Read the model definition and answer for the solid it produces. Units are mm, in the model's axes. Face numbers are marked on the shaded views. Round coordinates to 2 decimals unless told otherwise and drop trailing zeros. Loops run counter-clockwise (first coordinate to the right, second up) from the corner with the lowest first, then second, coordinate; pieces in that order, holes last. Notation, with made-up numbers: M 82.5,-30.75 L 91.5,-30.75 A37 ccw 91.5,5.25 Z; hole C 70.25,65.25 d1. An arc over 180 degrees is marked long. Write each question's results on one line, items separated by ' | '.
```python
from build123d import *

# Parameters (mm, degrees)
F0_R        = 1.075
F3_DEPTH    = 1.2
F2_W        = 15
F2_H        = 1.2
F4_DEPTH    = 10
F1_W        = 15
F1_H        = 1.2
F5_DEPTH    = 12
F6_T1_DEPTH = 38.762491
F7_R        = 2
F8_R        = 1
F10_D       = 3


# Not quite as in the source:
# - a fillet or chamfer that OpenCascade refuses, or shapes differently, is made with other operations: its cross-section is extruded or revolved along the edge and cut away or added


with BuildPart() as f3:
    # F0 (on Top) → F3 (new body)
    with BuildSketch(Plane.XY):
        Polygon((-15, 0), (0, 0), (0, 60), (-15, 60), (-15, 58.8), (-11, 58.8), (-10.4650629229, 8.8028616587), (-15, 7), align=None)
        with Locations((-2, 10)):
            Circle(F0_R, mode=Mode.SUBTRACT)
        with Locations((-2, 50)):
            Circle(F0_R, mode=Mode.SUBTRACT)
    extrude(amount=F3_DEPTH)

    # F2 (on face) → F4 (join)
    with BuildSketch(Plane.XY):
        with Locations((-7.5, 0.6)):
            Rectangle(F2_W, F2_H)
    extrude(amount=F4_DEPTH)

    # F1 (on face) → F5 (join)
    with BuildSketch(Plane.XY):
        with Locations((-7.5, 59.3886146865)):
            Rectangle(F1_W, F1_H)
    extrude(amount=F5_DEPTH)

    # F6: fillet of radius 7.5124982 on 2 edges, made by hand

    # F6_s2 → F6_t1 (cut)
    with BuildSketch(Plane.XZ.offset(-78.7698601865)):
        with BuildLine():
            ThreePointArc((0, 4.4875018), (-2.2003597791, 9.7996402209), (-7.5124982, 12))
            Line((-7.5124982, 12), (0, 12))
            Line((0, 12), (0, 4.4875018))
        make_face()
        with BuildLine():
            ThreePointArc((-15, 4.4875018), (-12.7996402209, 9.7996402209), (-7.4875018, 12))
            Line((-7.4875018, 12), (-15, 12))
            Line((-15, 12), (-15, 4.4875018))
        make_face()
    extrude(amount=F6_T1_DEPTH, mode=Mode.SUBTRACT)

    # F7
    f7_edges = [f3.edges().sort_by_distance(p)[0] for p in [
        (0, 0.6, 10),
        (-15, 0.6, 10),
    ]]
    fillet(f7_edges, radius=F7_R)

    # F8
    f8_edges = [f3.edges().sort_by_distance(p)[0] for p in [
        (-7.5, 0, 0),
        (-7.5, 60, 0),
    ]]
    fillet(f8_edges, radius=F8_R)

    # F10 (through all)
    with Locations(Plane.XZ):
        with Locations((-7.506201975, 4.490504507)):
            Hole(F10_D / 2)


solid = f3.part
```
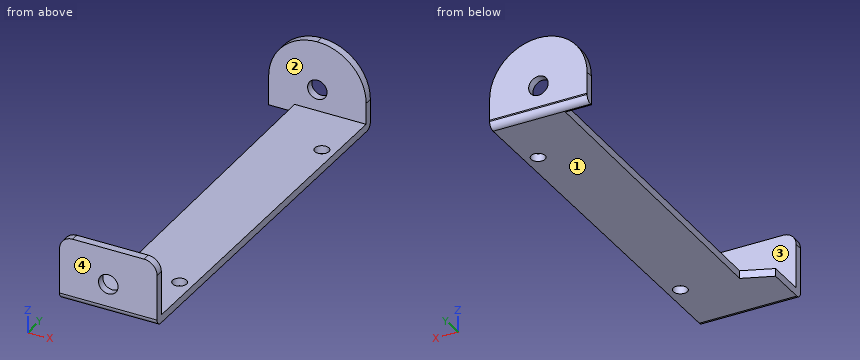
1. Given P1, Ø1, axis at x = -10.5, y = 24, coming from the +Z side; P2, Ø1, axis at x = -10, y = 1, coming from the +Z side; P3, Ø2.5, axis at x = -7.51, z = 4.49, coming from the -Y side; P4, Ø1, axis at x = -6.5, z = 5.5, coming from the +Y side, each flat-ended and moving along its own axis, determine where each tip first touches the part or whether it passes through.
Completed:
P1: stops at z = 1.2 | P2: stops at z = 10 | P3: passes through | P4: stops at y = 59.99
2. Find the intervals of material crossed by L1, parallel to Y at x = -2.75, z = 3; L2, parallel to Y at x = -2, z = 0.8 (3 decimals); L3, parallel to Y at x = -2, z = 0.4 (3 decimals), in increasing order.
Completed:
L1: y = 0 to 1.2, 58.79 to 59.99 | L2: y = 0.02 to 8.925, 11.075 to 48.925, 51.075 to 59.98 | L3: y = 0.2 to 8.925, 11.075 to 48.925, 51.075 to 59.8
3. Determine the mould class of the marked faces 1, 2, 3 and 4 for opening direction Y: released by +Y, released by -Y, zero draft, split by the parting line, or undercut.
Completed:
face 1: zero draft | face 2: undercut | face 3: undercut | face 4: released by -Y
4. Find section A-A, the plane z = 1.75. Give the vertices of the cut face in (x, y).
Completed:
outline: M -15,0 L 0,0 L 0,1.2 L -15,1.2 Z; M -15,58.79 L 0,58.79 L 0,59.99 L -15,59.99 Z
5. Find section B-B, the plane y = 10. Give the vertices of the cut face in (x, z) (3 decimals), then the cut area to 3 significant figures.
Completed:
outline: M -10.478,0 L -3.075,0 L -3.075,1.2 L -10.478,1.2 Z; M -0.925,0 L 0,0 L 0,1.2 L -0.925,1.2 Z | area: 9.99 mm2
6. Find section C-C, the plane z = 5.25. Give the vertices of the cut face in (x, y), then the cut area to 3 significant figures.
Completed:
outline: M -15,0 L -8.8,0 L -8.8,1.2 L -15,1.2 Z; M -14.96,58.79 L -8.8,58.79 L -8.8,59.99 L -14.96,59.99 Z; M -6.21,0 L 0,0 L 0,1.2 L -6.21,1.2 Z; M -6.21,58.79 L -0.04,58.79 L -0.04,59.99 L -6.21,59.99 Z | area: 29.7 mm2
